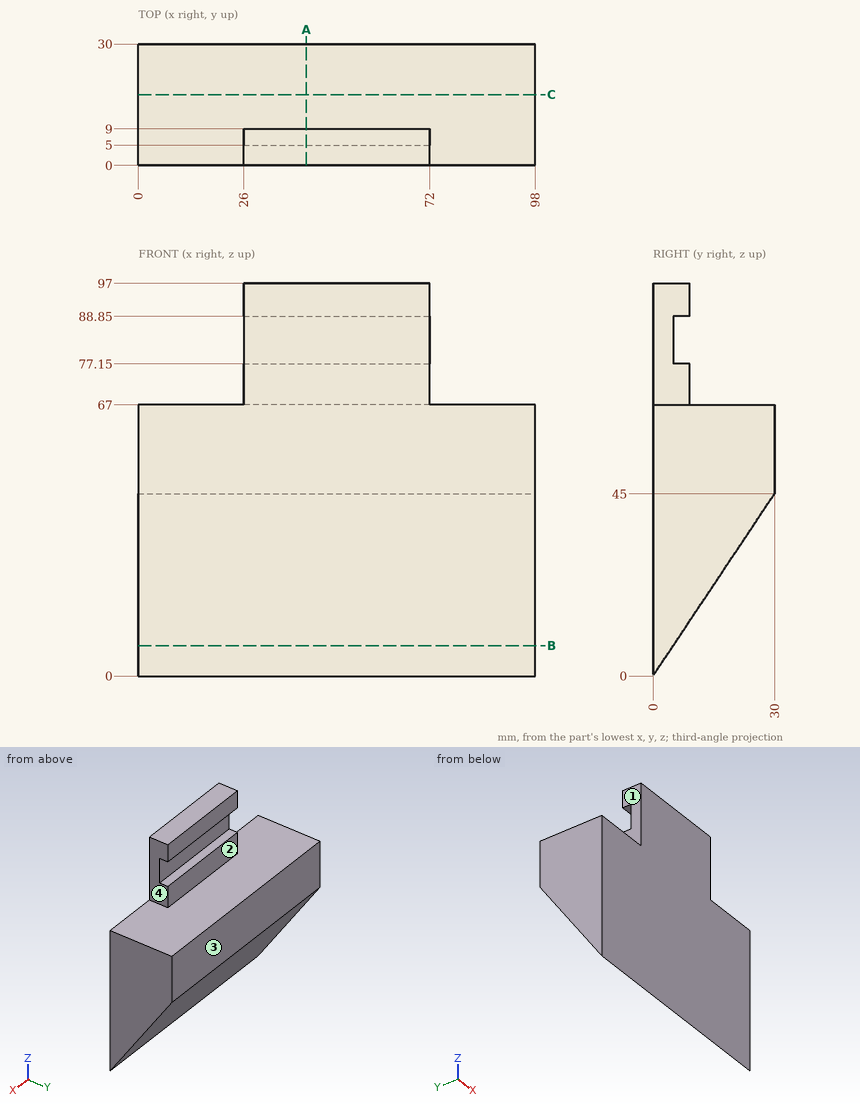
Part print with two shaded views. Sizes in mm from the minimum x, y, z corner. A direction names the side the tool comes from. Round coordinates to 2 decimals unless told otherwise and drop trailing zeros. Loops run counter-clockwise (first coordinate to the right, second up) from the corner with the lowest first, then second, coordinate; pieces in that order, holes last.
Item 1: Saw through at A-A (x = 41.5). List the corners of the cut face in (y, z), then the cut area to 3 significant figures.
Item 2: Drill centre lines: line 1 along Y through (x, z) = (66.5, 85.5); line 2 along Z through (x, y) = (69.5, 22); line 3 along Z through (x, y) = (76, 9.75) (3 decimals). Where is each one in solid material? Low to high.
Item 3: Saw through at C-C (y = 17.5). List the corners of the cut face in (x, z).
Item 4: Which spindle directions (+Z, -Z, +X, -X, +Y, -Y) get a long thin tool onto all of the face, cutting with end or side? Do the marked faces 1, 2, 3 and 4. Say none if no direction does.
Item 5: Pin check, flat tips, straight feed: P1, Ø1.5, axis at x = 57.5, y = 4, coming from the -Z side (3 decimals); P2, Ø7, axis at y = 3, z = 84, coming from the +X side; P3, Ø2.5, axis at y = 3.5, z = 81, coming from the -X side. Stop position of each tip, or through.
Item 6: Saw through at B-B (z = 7.5). List the corners of the cut face in (x, y), then the cut area to 3 significant figures.
Worked answers:
1. outline: (0, 0) - (30, 45) - (30, 67) - (9, 67) - (9, 77.15) - (5, 77.15) - (5, 88.85) - (9, 88.85) - (9, 97) - (0, 97) - close
1. area: 1,560 mm2
2. line 1: y = 0 to 5
2. line 2: z = 33 to 67
2. line 3: z = 14.625 to 67
3. outline: (0, 26.25) - (98, 26.25) - (98, 67) - (0, 67) - close
4. face 1: +Z, -X, +Y, -Y
4. face 2: +Z, +X, -X, +Y
4. face 3: +Z, -Z, +X, -X, +Y
4. face 4: +Z, +X, +Y, -Y
5. P1: stops at z = 4.875
5. P2: stops at x = 72
5. P3: stops at x = 26
6. outline: (0, 0) - (98, 0) - (98, 5) - (0, 5) - close
6. area: 490 mm2
